```python
from build123d import *

# Parameters (mm, degrees)
EXTRUDE_1_DEPTH     = 3
SKETCH_2_R          = 2.1
CUT_EXTRUDE_1_DEPTH = 39
FILLET_1_R          = 4


with BuildPart() as part:
    # Эскиз1 → Бобышка-Вытянуть1 (new body)
    with BuildSketch(Plane.XY):
        Polygon((0, 0), (0, 140), (230, -20), (230, -60), (200, -60), align=None)
    extrude(amount=EXTRUDE_1_DEPTH)

    # Эскиз2 → Вырез-Вытянуть1 (cut)
    with BuildSketch(Plane.XY.offset(3)):
        with Locations((10, 74)):
            Circle(SKETCH_2_R)
        with Locations((10, 119.2)):
            Circle(SKETCH_2_R)
    extrude(amount=-CUT_EXTRUDE_1_DEPTH, mode=Mode.SUBTRACT)

    # Скругление1
    fillet_1_edges = [part.edges().sort_by_distance(p)[0] for p in [
        (0, 0, 1.5),
        (0, 140, 1.5),
        (230, -20, 1.5),
        (230, -60, 1.5),
        (200, -60, 1.5),
    ]]
    fillet(fillet_1_edges, radius=FILLET_1_R)


solid = part.part
```
Check sheet for the modelled part. Datum: model origin and axes. Units: mm. Coordinates: 2 decimals unless noted, no trailing zeros. Loops run counter-clockwise (first coordinate to the right, second up) from the corner with the lowest first, then second, coordinate; pieces in that order, holes last.
1) Gauge pin test, flat ends, axial feed: pin 1 (1.5 mm diameter, centred on x = 192, z = 2.5, fed in from +Y); pin 2 (2.5 mm diameter, centred on x = 10, y = 119.2, fed in from -Z); pin 3 (1 mm diameter, centred on x = 163.5, z = 1.5, fed in from +Y). Record the tip position at first contact, or that the pin passes through.
2) Material ranges on probe 1 along Y at (x, z) = (10, 0.9); probe 2 along Y at (x, z) = (177, 1.7); probe 3 along X at (y, z) = (86, 0.3) (3 decimals), recorded low to high.
3) Sectioned sample at B-B (x = 23). Record the boundary of the cut face in (y, z).
4) Sectioned sample at A-A (z = 0.85). Record the boundary of the cut face in (x, y).
5) Sectioned sample at C-C (y = 14). Record the boundary of the cut face in (x, z) (3 decimals), and give its area (3 significant figures).
Check sheet entries:
1. pin 1: stops at y = 6.96
1. pin 2: passes through
1. pin 3: stops at y = 26.61
2. probe 1: y = -3 to 71.9, 76.1 to 117.1, 121.3 to 133.04
2. probe 2: y = -53.1 to 16.87
2. probe 3: x = 0 to 77.625
3. outline: (-6.9, 0) - (124, 0) - (124, 3) - (-6.9, 3) - close
4. outline: (0, 2.98) arc R4 ccw to (2.85, -0.86) - (199.44, -59.83) arc R4 ccw to (200.59, -60) - (226, -60) arc R4 ccw to (230, -56) - (230, -22.09) arc R4 ccw to (228.28, -18.81) - (6.28, 135.63) arc R4 ccw to (0, 132.34) - close; hole circle Ø4.2 at (10, 74); hole circle Ø4.2 at (10, 119.2)
5. outline: (0, 0) - (181.125, 0) - (181.125, 3) - (0, 3) - close
5. area: 543 mm2
